from build123d import *

# Parameters (mm, degrees)
SKETCH4_W          = 1.2
SKETCH4_H          = 1.2
CUT_EXTRUDE2_DEPTH = 29.526829477
CIRPATTERN1_COUNT  = 10


with BuildPart() as part:
    # Sketch1 → Revolve1 (revolve)
    with BuildSketch(Plane.XY, mode=Mode.PRIVATE) as revolve1_sk:
        Polygon((-7.2, -4), (-7.2, 12), (-8, 12), (-8, 0), (-17.5, 0), (-17.5, 12), (-18.3, 12), (-18.3, -8), (-4.3, -8), (-4.3, -4), align=None)
    revolve(revolve1_sk.sketch.rotate(Axis((0, 0, 0), (0, -1, 0)), 270), axis=Axis((0, 0, 0), (0, -1, 0)))

    # Sketch4 → Cut-Extrude2 (cut, through all)
    with BuildSketch(Plane(origin=(0, 0, 0), x_dir=(0, 0, -1), z_dir=(1, 0, 0))):
        with Locations((0, 11.4)):
            Rectangle(SKETCH4_W, SKETCH4_H)
    cut_extrude2 = extrude(amount=-CUT_EXTRUDE2_DEPTH, mode=Mode.SUBTRACT)

    # CirPattern1: Cut-Extrude2 ×10 about axis
    cirpattern1_axis = Axis((0, 0, 0), (0, 1, 0))
    for i in range(1, CIRPATTERN1_COUNT):
        add(cut_extrude2.rotate(cirpattern1_axis, i * 360 / CIRPATTERN1_COUNT), mode=Mode.SUBTRACT)


solid = part.part
Verification items for the finished model (mm, model axes). A direction names the side the tool comes from. Give positions to 0.01 mm unless a question says otherwise; leave off trailing zeros. Loops run counter-clockwise (first coordinate to the right, second up) from the corner with the lowest first, then second, coordinate; pieces in that order, holes last.
1) Set-up check for faces 3 (the flat face through (-7.1, 12, -2.4)), 4 (the flat face through (-6.1, 10.8, 4.5)): record each of +Z, -Z, +X, -X, +Y, -Y from which the full face is reachable in a straight line by a thin tool's end or side.
2) Draft check along X on faces 1 (the flat face through (-14.5, 10.8, -10.5)), 2 (the flat face through (-17, 12, -5)). Enter one of: pulls with the +X half, pulls with the -X half, needs draft (parallel to the pull), parting line crosses it, or undercut.
3) Sectioned sample at B-B, the plane z = 0. Enter the section's corners in (x, y), then the cut area to 3 significant figures.
4) Sectioned sample at C-C, the plane y = 3.25. Enter the section's corners in (x, z).
5) Sectioned sample at A-A, the plane x = 0. Enter the section's corners in (y, z), then the cut area to 3 significant figures.
6) Sectioned sample at D-D, the plane y = -1.75. Enter the section's corners in (x, z), then the cut area to 3 significant figures.
7) Depth check by flat-ended pin: pin 1 Ø2 at (y, z) = (7, -5.5) entering from -X; pin 2 Ø1.5 at (x, z) = (6.5, -4.5) entering from +Y; pin 3 Ø12 at (y, z) = (9, 10.5) entering from +X; pin 4 Ø4 at (y, z) = (-3, 5) entering from +X. Enter the tip coordinate at first touch or a pass-through.
8) Thickness scan on line 1 along X through (y, z) = (1.25, 0); line 2 along X through (y, z) = (-6.95, 0); line 3 along X through (y, z) = (9.5, -5.5). Record the ranges inside material, lowest first.
Answers:
1. face 3: +Z, -Z, +X, -X, +Y
1. face 4: +Y
2. face 1: undercut
2. face 2: needs draft
3. outline: (-18.3, -8) - (-4.3, -8) - (-4.3, -4) - (-7.2, -4) - (-7.2, 10.8) - (-8, 10.8) - (-8, 0) - (-17.5, 0) - (-17.5, 10.8) - (-18.3, 10.8) - close; (4.3, -8) - (18.3, -8) - (18.3, 10.8) - (17.5, 10.8) - (17.5, 0) - (8, 0) - (8, 10.8) - (7.2, 10.8) - (7.2, -4) - (4.3, -4) - close
3. area: 235 mm2
4. outline: circle Ø36.6 at (0, 0); circle Ø16 at (0, 0); hole circle Ø35 at (0, 0); hole circle Ø14.4 at (0, 0)
5. outline: (-8, -18.3) - (12, -18.3) - (12, -17.5) - (0, -17.5) - (0, -8) - (12, -8) - (12, -7.2) - (-4, -7.2) - (-4, -4.3) - (-8, -4.3) - close; (-8, 4.3) - (-4, 4.3) - (-4, 7.2) - (12, 7.2) - (12, 8) - (0, 8) - (0, 17.5) - (12, 17.5) - (12, 18.3) - (-8, 18.3) - close
5. area: 239 mm2
6. outline: circle Ø36.6 at (0, 0); hole circle Ø14.4 at (0, 0)
6. area: 889 mm2
7. pin 1: stops at x = -17.74
7. pin 2: stops at y = 12
7. pin 3: stops at x = 17.74
7. pin 4: stops at x = 18.05
8. line 1: x = -18.3 to -17.5, -8 to -7.2, 7.2 to 8, 17.5 to 18.3
8. line 2: x = -18.3 to -4.3, 4.3 to 18.3
8. line 3: x = -17.45 to -16.61, -5.81 to -4.65, 4.65 to 5.81, 16.61 to 17.45
